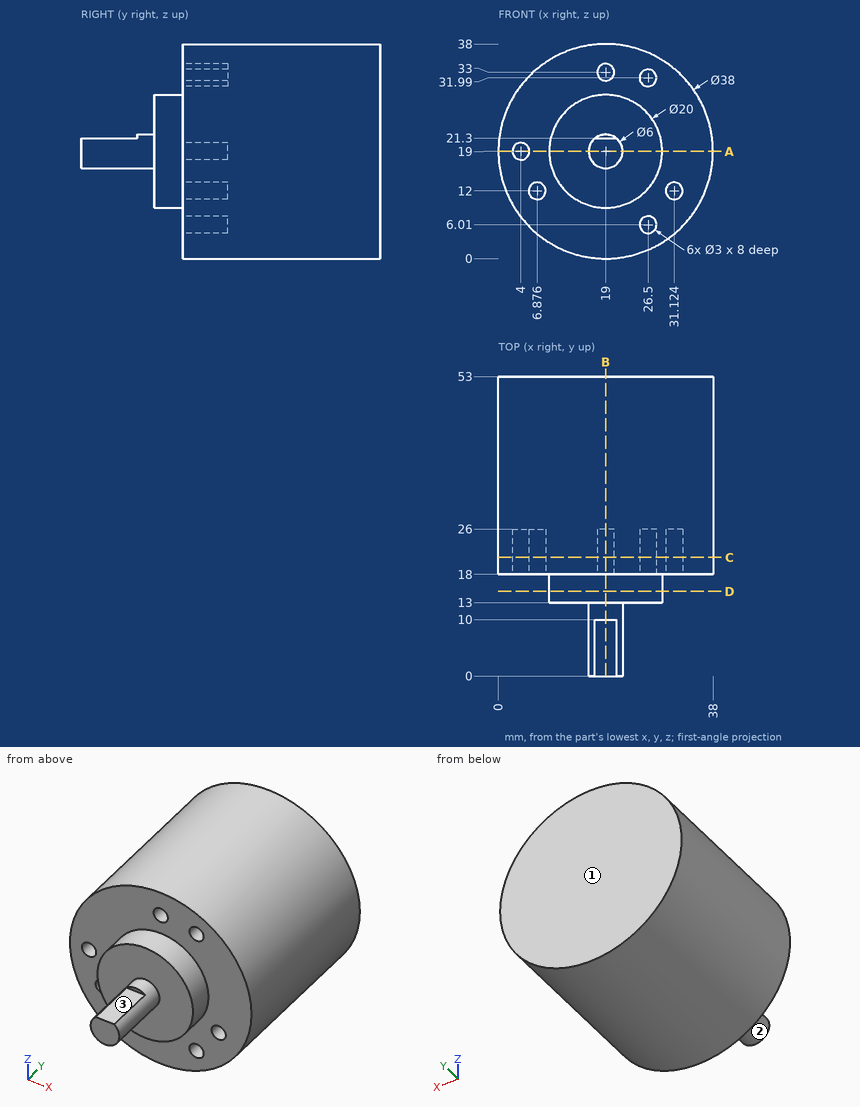
Here's the drawing with two shaded views (mm, measured from the low corner). I have some questions. A direction names the side the tool comes from. Give positions to 0.01 mm unless a question says otherwise; leave off trailing zeros. Order: outer loops, then holes, each group sorted by start corner. A loop starts at its lowest first (then second) coordinate and runs counter-clockwise, first axis right, second up. Notation, with made-up numbers: (-20.5, -14) -> (-8.5, -14) arc R19 ccw to (-8.5, -10) -> close; hole circle Ø1 at (-39.5, 26.25). An arc over 180 degrees is marked (long way). One line per item, written item: value. Start each with the question number.
1. Imagine slicing it at B-B, the plane x = 19. List the corners of the cut face in (y, z) for me.
2. Imagine slicing it at C-C, the plane y = 21. Count the separate pieces of the cut face and the enclosed holes in it, plus the area to 3 significant figures.
3. Will these pins go through, and if not, where does the flat tip stop? pin 1 Ø1.5 at (x, z) = (26.5, 5.5) entering from -Y; pin 2 Ø12 at (y, z) = (47.5, 6) entering from +X; pin 3 Ø2 at (y, z) = (12.5, 13.5) entering from -X.
4. Imagine slicing it at D-D, the plane y = 15. List the corners of the cut face in (x, z) for me.
5. Imagine slicing it at A-A, the plane z = 19. List the corners of the cut face in (x, y) for me, plus the area to 3 significant figures.
6. For the marked faces 1, 2 and 3, which set-ups out of +Z, -Z, +X, -X, +Y, -Y let a thin tool reach every point of the face, with its end or its side?
7. I need wall thicknesses on probe 1 along Z at (x, y) = (27.5, 18.5); probe 2 along Z at (x, y) = (26.5, 23); probe 3 along Y at (x, z) = (11, 3.5). Which ranges of each line are inside material? Lowest first, please. Write a range as from..to.
Values follow:
1. outline: (0, 16) -> (13, 16) -> (13, 9) -> (18, 9) -> (18, 0) -> (53, 0) -> (53, 38) -> (18, 38) -> (18, 34.5) -> (26, 34.5) -> (26, 31.5) -> (18, 31.5) -> (18, 29) -> (13, 29) -> (13, 22) -> (10, 22) -> (10, 21.3) -> (0, 21.3) -> close
2. separate pieces: 1
2. enclosed holes: 6
2. area: 1,090 mm2
3. pin 1: stops at y = 26
3. pin 2: stops at x = 36.66
3. pin 3: stops at x = 10.14
4. outline: circle Ø20 at (19, 19)
5. outline: (0, 18) -> (2.5, 18) -> (2.5, 26) -> (5.5, 26) -> (5.5, 18) -> (9, 18) -> (9, 13) -> (16, 13) -> (16, 0) -> (22, 0) -> (22, 13) -> (29, 13) -> (29, 18) -> (38, 18) -> (38, 53) -> (0, 53) -> close
5. area: 1,480 mm2
6. face 1: +Z, -Z, +X, -X, +Y
6. face 2: -Y
6. face 3: +Z, +X, -X, -Y
7. probe 1: z = 2.01..4.89, 7.13..30.87, 33.11..35.99
7. probe 2: z = 1.54..4.51, 7.51..30.49, 33.49..36.46
7. probe 3: y = 18..53
